Check sheet for the modelled part. Datum: model origin and axes. Units: mm. A direction names the side the tool comes from. Round coordinates to 2 decimals unless told otherwise and drop trailing zeros. Loops run counter-clockwise (first coordinate to the right, second up) from the corner with the lowest first, then second, coordinate; pieces in that order, holes last. Notation, with made-up numbers: (-13, 65) -> (38, 65) arc R11 cw to (38, 86) -> close; hole circle Ø5 at (-32.5, 47). An arc over 180 degrees is marked (long way). One line per item, written item: value. Start each with the question number.
1. Go/stop test with flat-tipped pins: pin 1 (4 mm diameter, centred on x = 12.5, y = 25.5, fed in from +Z); pin 2 (6 mm diameter, centred on x = -9, z = 70, fed in from +Y); pin 3 (6 mm diameter, centred on x = 28.5, z = -17.5, fed in from -Y); pin 4 (8 mm diameter, centred on x = -6, z = 44, fed in from +Y). Record where each tip stops, or that it passes through.
2. Material ranges on L1, parallel to X at y = 1, z = -6; L2, parallel to X at y = 3.2, z = -94.1, recorded low to high.
3. Set-up check for faces 1 (the face through (2.6, 31, -25.1)), 2 (the face through (-10, 5, 62)), 3 (the face through (-10, 5, -83)): record each of +Z, -Z, +X, -X, +Y, -Y from which the full face is reachable in a straight line by a thin tool's end or side.
4. Release check for a two-part mould opening along X. For faces 4 (the face through (2.5, 31, 5)), 5 (the face through (0, 12, -47)), 6 (the face through (-10, 24, 0)), 7 (the face through (-100.1, 2, -10)) record: +X half, -X half, draft (parallel to the pull), parting line (faces both ways), or undercut.
5. Cross-section at B-B on z = 55. Record the cut outline in (x, y).
6. Cross-section at A-A on x = 63. Record the cut outline in (y, z).
from build123d import *

# Parameters (mm, degrees)
SKETCH1_W             = 75
SKETCH1_H             = 20.1
SKETCH1_R             = 1.55
BOSS_EXTRUDE1_DEPTH   = 5
SKETCH1_W_2           = 20.1
SKETCH1_H_2           = 75
BOSS_EXTRUDE1_2_DEPTH = 5
BOSS_EXTRUDE1_3_DEPTH = 5
BOSS_EXTRUDE1_4_DEPTH = 5
SKETCH1_8_W           = 5
SKETCH1_8_H           = 5
SKETCH1_8_W_2         = 20.1
SKETCH1_8_H_2         = 20.1
BOSS_EXTRUDE2_DEPTH   = 50
CHAMFER1_SIZE         = 40
FILLET1_R             = 2


with BuildPart() as part:
    # Sketch1 → Boss-Extrude1 (new body)
    with BuildSketch(Plane(origin=(0, 0, 0), x_dir=(1, 0, 0), z_dir=(0, 1, 0))):
        with Locations((42.5, 10.05)):
            Rectangle(SKETCH1_W, SKETCH1_H)
        with Locations((74, 6)):
            Circle(SKETCH1_R, mode=Mode.SUBTRACT)
        with Locations((74, 14.1)):
            Circle(SKETCH1_R, mode=Mode.SUBTRACT)
    extrude(amount=BOSS_EXTRUDE1_DEPTH)



with BuildPart() as body_2:
    # Sketch1 → Boss-Extrude1 2 (new body)
    with BuildSketch(Plane(origin=(0, 0, 0), x_dir=(1, 0, 0), z_dir=(0, 1, 0))):
        with Locations((-10.05, -42.5)):
            Rectangle(SKETCH1_W_2, SKETCH1_H_2)
        with Locations((-14.1, -74)):
            Circle(SKETCH1_R, mode=Mode.SUBTRACT)
        with Locations((-6, -74)):
            Circle(SKETCH1_R, mode=Mode.SUBTRACT)
    extrude(amount=BOSS_EXTRUDE1_2_DEPTH)


with BuildPart() as body_3:
    # Sketch1 → Boss-Extrude1 3 (new body)
    with BuildSketch(Plane(origin=(0, 0, 0), x_dir=(1, 0, 0), z_dir=(0, 1, 0))):
        with Locations((-10.05, 62.6)):
            Rectangle(SKETCH1_W_2, SKETCH1_H_2)
        with Locations((-14.1, 94.1)):
            Circle(SKETCH1_R, mode=Mode.SUBTRACT)
        with Locations((-6, 94.1)):
            Circle(SKETCH1_R, mode=Mode.SUBTRACT)
    extrude(amount=BOSS_EXTRUDE1_3_DEPTH)


with BuildPart() as body_4:
    # Sketch1 → Boss-Extrude1 4 (new body)
    with BuildSketch(Plane(origin=(0, 0, 0), x_dir=(1, 0, 0), z_dir=(0, 1, 0))):
        with Locations((-62.6, 10.05)):
            Rectangle(SKETCH1_W, SKETCH1_H)
        with Locations((-94.1, 6)):
            Circle(SKETCH1_R, mode=Mode.SUBTRACT)
        with Locations((-94.1, 14.1)):
            Circle(SKETCH1_R, mode=Mode.SUBTRACT)
    extrude(amount=BOSS_EXTRUDE1_4_DEPTH)


with BuildPart() as part_1:
    add(part.part)

    add(body_2.part)  # Boss-Extrude2 merges body 2

    add(body_3.part)  # Boss-Extrude2 merges body 3

    add(body_4.part)  # Boss-Extrude2 merges body 4
    # Sketch1_8 → Boss-Extrude2 (add)
    with BuildSketch(Plane(origin=(0, 0, 0), x_dir=(1, 0, 0), z_dir=(0, 1, 0))):
        with Locations((-22.6, 22.6)):
            Rectangle(SKETCH1_8_W, SKETCH1_8_H)
        with Locations((-10.05, 22.6)):
            Rectangle(SKETCH1_8_W_2, SKETCH1_8_H)
        with Locations((-22.6, 10.05)):
            Rectangle(SKETCH1_8_W, SKETCH1_8_H_2)
        with Locations((2.5, 22.6)):
            Rectangle(SKETCH1_8_W, SKETCH1_8_H)
        with Locations((2.5, 10.05)):
            Rectangle(SKETCH1_8_W, SKETCH1_8_H_2)
        with Locations((2.5, -2.5)):
            Rectangle(SKETCH1_8_W, SKETCH1_8_H)
        with Locations((-10.05, -2.5)):
            Rectangle(SKETCH1_8_W_2, SKETCH1_8_H)
        with Locations((-22.6, -2.5)):
            Rectangle(SKETCH1_8_W, SKETCH1_8_H)
    extrude(amount=BOSS_EXTRUDE2_DEPTH)

    # Chamfer1
    chamfer1_edges = [part_1.edges().sort_by_distance(p)[0] for p in [
        (5, 5, -10.05),
        (-10.05, 5, -25.1),
        (-25.1, 5, -10.05),
        (-10.05, 5, 5),
    ]]
    chamfer(chamfer1_edges, length=CHAMFER1_SIZE)

    # Fillet1
    fillet1_edges = [part_1.edges().sort_by_distance(p)[0] for p in [
        (5, 25, 0),
        (5, 25, -20.1),
        (5, 50, -10.05),
        (5, 25, 5),
        (0, 50, -10.05),
        (0, 25, -20.1),
        (-10.05, 50, 0),
        (0, 25, 0),
        (-20.1, 50, -10.05),
        (-20.1, 25, 0),
        (-25.1, 25, 5),
        (-10.05, 50, -25.1),
        (5, 25, -25.1),
        (-25.1, 25, -25.1),
        (-20.1, 25, -20.1),
        (-10.05, 50, 5),
        (-25.1, 50, -10.05),
        (-10.05, 50, -20.1),
        (-20.1, 25, -25.1),
        (0, 25, -25.1),
        (-25.1, 25, 0),
        (-25.1, 25, -20.1),
        (0, 25, 5),
        (-20.1, 25, 5),
        (-10.05, 45, -25.1),
        (5, 45, -10.05),
        (-10.05, 45, 5),
        (-25.1, 45, -10.05),
    ]]
    fillet(fillet1_edges, radius=FILLET1_R)


solid = part_1.part
Taken from the geometry:
1. pin 1: stops at z = 0
1. pin 2: stops at y = 5
1. pin 3: stops at y = 0
1. pin 4: stops at y = 10
2. L1: x = -100.1 to -95.65, -92.55 to -20.1, 0 to 72.45, 75.55 to 80
2. L2: x = -20.1 to -15.65, -12.55 to -7.55, -4.45 to 0
3. face 1: -Z, +Y
3. face 2: +Z, +X, -X, +Y
3. face 3: -Z, +X, -X, +Y
4. face 4: draft
4. face 5: +X half
4. face 6: undercut
4. face 7: -X half
5. outline: (-20.1, 0) -> (0, 0) -> (0, 5) -> (-20.1, 5) -> close
6. outline: (0, -20.1) -> (5, -20.1) -> (5, 0) -> (0, 0) -> close
